Design review of the part built by this model. Coordinates are the model's own, in mm. Coordinates: 2 decimals unless noted, no trailing zeros. Loops run counter-clockwise (first coordinate to the right, second up) from the corner with the lowest first, then second, coordinate; pieces in that order, holes last. Notation, with made-up numbers: M 50,-1 L 72,-1 A7 ccw 72,3 Z; hole C 72,73 d7. An arc over 180 degrees is marked long. Answer as a JSON object with one key per item and string values. Group by question number.
1. Consider section C-C (y = 1.5). State the section outline as (x, z) points, then the cut area to 3 significant figures.
2. To check wall thickness, follow probe 1 along X at (y, z) = (7.25, 2.1); probe 2 along Y at (x, z) = (30.5, 0.3); probe 3 along Z at (x, y) = (36.5, 11). State the ranges of each line that lie inside material, in increasing order.
3. Insertion check: pin 1 (0.6 mm diameter, centred on y = 7, z = 1.5, fed in from +X); pin 2 (0.6 mm diameter, centred on x = 18.5, y = 5.5, fed in from +Z); pin 3 (1.1 mm diameter, centred on x = 18.5, z = 1, fed in from -Y). Each pin has a flat end and moves straight along its axis. Give the tip position at first contact, or say it passes through.
4. Consider section B-B (z = 1.2). Count the separate pieces of the cut face and the enclosed holes in it, then the cut area to 3 significant figures.
5. Consider section A-A (y = -2.25). State the section outline as (x, z) points (3 decimals).
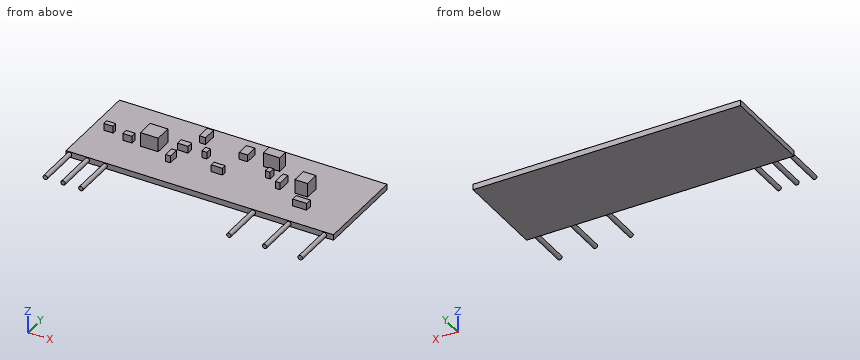
from build123d import *

# Parameters (mm, degrees)
ESQUISSE1_W        = 38.1
ESQUISSE1_H        = 13.2
BOSS_EXTRU_1_DEPTH = 0.8
ESQUISSE2_R        = 0.315
BOSS_EXTRU_2_DEPTH = 6
ESQUISSE3_W        = 2.528787401
ESQUISSE3_H        = 2.40642672
ESQUISSE3_W_2      = 2.324852932
ESQUISSE3_H_2      = 1.468328168
ESQUISSE3_W_3      = 1.794623316
ESQUISSE3_H_3      = 2.080131572
BOSS_EXTRU_3_DEPTH = 2
ESQUISSE4_W        = 1.288030783
ESQUISSE4_H        = 0.792634328
ESQUISSE4_H_2      = 0.693555037
ESQUISSE4_W_2      = 0.693555037
ESQUISSE4_H_3      = 1.486189366
ESQUISSE4_W_3      = 1.486189365
ESQUISSE4_H_4      = 0.891713619
ESQUISSE4_W_4      = 1.585268657
ESQUISSE4_W_5      = 0.891713619
ESQUISSE4_H_5      = 1.981585821
ESQUISSE4_W_6      = 1.188951492
ESQUISSE4_H_6      = 1.783427238
ESQUISSE4_H_7      = 1.932046175
ESQUISSE4_W_7      = 1.98158582
BOSS_EXTRU_8_DEPTH = 1


with BuildPart() as part:
    # Esquisse1 → Boss.-Extru.1 (new body)
    with BuildSketch(Plane.XY):
        with Locations((19.05, 6.6)):
            Rectangle(ESQUISSE1_W, ESQUISSE1_H)
    extrude(amount=BOSS_EXTRU_1_DEPTH)

    # Esquisse2 → Boss.-Extru.2 (add)
    with BuildSketch(Plane.XZ):
        with Locations(Location((0.5, 0.399671485, 0), (0, 0, 90))):
            Circle(ESQUISSE2_R)
        with Locations(Location((3.04, 0.399671485, 0), (0, 0, 90))):
            Circle(ESQUISSE2_R)
        with Locations(Location((5.58, 0.399671485, 0), (0, 0, 90))):
            Circle(ESQUISSE2_R)
        with Locations(Location((26.67, 0.399671485, 0), (0, 0, 90))):
            Circle(ESQUISSE2_R)
        with Locations(Location((31.75, 0.399671485, 0), (0, 0, 90))):
            Circle(ESQUISSE2_R)
        with Locations(Location((36.83, 0.399671485, 0), (0, 0, 90))):
            Circle(ESQUISSE2_R)
    extrude(amount=BOSS_EXTRU_2_DEPTH)

    # Esquisse3 → Boss.-Extru.3 (add)
    with BuildSketch(Plane.XY.offset(0.8)):
        with Locations((8.710522484, 6.659017017)):
            Rectangle(ESQUISSE3_W, ESQUISSE3_H)
        with Locations((24.026001014, 9.820001267)):
            Rectangle(ESQUISSE3_W_2, ESQUISSE3_H_2)
        with Locations((30.164428494, 6.822164591)):
            Rectangle(ESQUISSE3_W_3, ESQUISSE3_H_3)
    extrude(amount=BOSS_EXTRU_3_DEPTH)

    # Esquisse4 → Boss.-Extru.8 (add)
    with BuildSketch(Plane.XY.offset(0.8)):
        with Locations((5.552416897, 5.933480073)):
            Rectangle(ESQUISSE4_W, ESQUISSE4_H)
        with Locations((2.381879584, 6.676574756)):
            Rectangle(ESQUISSE4_W, ESQUISSE4_H_2)
        with Locations((12.190729396, 4.794068226)):
            Rectangle(ESQUISSE4_W_2, ESQUISSE4_H_3)
        with Locations((12.58704656, 7.469209084)):
            Rectangle(ESQUISSE4_W_3, ESQUISSE4_H_4)
        with Locations((18.680422957, 5.190385391)):
            Rectangle(ESQUISSE4_W_4, ESQUISSE4_H_2)
        with Locations((15.658504582, 7.469209084)):
            Rectangle(ESQUISSE4_W_2, ESQUISSE4_H_4)
        with Locations((13.775998052, 10.788365333)):
            Rectangle(ESQUISSE4_W_5, ESQUISSE4_H_5)
        with Locations((20.067533032, 9.896651714)):
            Rectangle(ESQUISSE4_W_6, ESQUISSE4_H_6)
        with Locations((24.674720065, 7.469209084)):
            Rectangle(ESQUISSE4_W_2, ESQUISSE4_H_4)
        with Locations((26.953543759, 6.503185997)):
            Rectangle(ESQUISSE4_W_2, ESQUISSE4_H_7)
        with Locations((31.4616515, 3.605116734)):
            Rectangle(ESQUISSE4_W_7, ESQUISSE4_H_4)
    extrude(amount=BOSS_EXTRU_8_DEPTH)


solid = part.part
Findings below:
{
 "1": {"outline": "M 0,0 L 38.1,0 L 38.1,0.8 L 0,0.8 Z", "area": "30.5 mm^2"},
 "2": {"probe 1": "x = 7.45 to 9.97, 29.27 to 31.06", "probe 2": "y = 0 to 13.2", "probe 3": "z = 0 to 0.8"},
 "3": {"pin 1": "stops at x = 31.06", "pin 2": "stops at z = 1.8", "pin 3": "stops at y = 0"},
 "4": {"separate pieces": "14", "enclosed holes": "0", "area": "26.8 mm^2"},
 "5": {"outline": "C 0.5,0.4 d0.63; C 3.04,0.4 d0.63; C 5.58,0.4 d0.63; C 26.67,0.4 d0.63; C 31.75,0.4 d0.63; C 36.83,0.4 d0.63"}
}
